Verification items for the finished model (mm, model axes). A direction names the side the tool comes from. Give positions to 0.01 mm unless a question says otherwise; leave off trailing zeros. Order: outer loops, then holes, each group sorted by start corner. A loop starts at its lowest first (then second) coordinate and runs counter-clockwise, first axis right, second up. Notation, with made-up numbers: M 64.25,15 L 117.25,15 A15 cw 117.25,21 Z; hole C -33,69 d9. An arc over 180 degrees is marked long. Answer as a JSON object with one key per item and string values.
```python
from build123d import *

# Parameters (mm, degrees)
BOSS_EXTRUDE1_START = -60
BOSS_EXTRUDE1_DEPTH = 60


with BuildPart() as part:
    # Sketch1 → Boss-Extrude1 (new body)
    with BuildSketch(Plane.XY.offset(BOSS_EXTRUDE1_START)):
        with BuildLine():
            ThreePointArc((34.60288698, -49.016734007), (30, -51.961524227), (25.14829337, -54.475346172))
            Line((25.14829337, -54.475346172), (27.613812707, -61.249304876))
            ThreePointArc((27.613812707, -61.249304876), (27.55707569, -63.445610174), (26.01881055, -65.014277255))
            ThreePointArc((26.01881055, -65.014277255), (34.999997878, -60.621774589), (43.294610437, -55.040089541))
            ThreePointArc((43.294610437, -55.040089541), (41.166972324, -55.587932689), (39.236547633, -54.538915737))
            Line((39.236547633, -54.538915737), (34.60288698, -49.016734007))
        make_face()
    extrude(amount=BOSS_EXTRUDE1_DEPTH)


solid = part.part
```
Q1. Material ranges on L1, parallel to Y at x = 34.75, z = -19.5; L2, parallel to X at y = -53, z = -45.5; L3, parallel to X at y = -56.75, z = -30, recorded low to high.
Resolved:
{"L1": "y = -60.77 to -49.19", "L2": "x = 28.12 to 37.95", "L3": "x = 25.98 to 41"}
Q2. Gauge pin test, flat ends, axial feed: pin 1 Ø4 at (x, z) = (39.5, -48) entering from -Y; pin 2 Ø5 at (x, z) = (41.5, -40) entering from +Y; pin 3 Ø4 at (x, z) = (30, -44) entering from -Y. Record the tip position at first contact, or that the pin passes through.
Resolved:
{"pin 1": "stops at y = -59.11", "pin 2": "stops at y = -54.26", "pin 3": "stops at y = -64.17"}
Q3. Tool access check on faces 5 (the face through (30.07, -51.92, -30.42)), 6 (the face through (26.36, -57.81, -30.42)). Record the directions out of +Z, -Z, +X, -X, +Y, -Y that give a thin tool (end or side, any length) a straight path to the whole face; none if there is none.
Resolved:
{"face 5": "+Z, -Z, -X, +Y", "face 6": "+Z, -Z, -X"}
Q4. Section check B-B on x = 40.5. Record the cut outline in (y, z), then the cut area to 3 significant figures.
Resolved:
{"outline": "M -57.11,-60 L -55.43,-60 L -55.43,0 L -57.11,0 Z", "area": "101 mm²"}
Q5. Section check C-C on y = -60.5. Record the cut outline in (x, z).
Resolved:
{"outline": "M 27.34,-60 L 35.21,-60 L 35.21,0 L 27.34,0 Z"}
Q6. Section check A-A on z = -33. Record the cut outline in (x, y).
Resolved:
{"outline": "M 25.15,-54.48 L 27.61,-61.25 A3 cw 26.02,-65.01 A72.79 ccw 43.29,-55.04 A3 cw 39.24,-54.54 L 34.6,-49.02 A60 cw Z"}
Q7. Release check for a two-part mould opening along Y. For faces 1 (the face through (27.569, -63.417, -30.42)), 2 (the face through (34.88, -60.69, -30.42)), 3 (the face through (32, -57, -60)), 4 (the face through (41.2, -55.59, -30.42)) record: +Y half, -Y half, draft (parallel to the pull), parting line (faces both ways), or undercut.
Resolved:
{"face 1": "undercut", "face 2": "-Y half", "face 3": "draft", "face 4": "+Y half"}
